Model file for the job. Use its own axes, mm. Face numbers are marked on the shaded views. A direction names the side the tool comes from. Round coordinates to 2 decimals unless told otherwise and drop trailing zeros. Loops run counter-clockwise (first coordinate to the right, second up) from the corner with the lowest first, then second, coordinate; pieces in that order, holes last. Notation, with made-up numbers: M -20.75,34.25 L 9.25,34.25 A24 ccw 9.25,62.25 Z; hole C -22,38 d9. An arc over 180 degrees is marked long. Use a Markdown table: item, result. Add a question column.
Item 1: Pin check, flat tips, straight feed: P1, Ø1, axis at x = 0.5, z = -1, coming from the +Y side; P2, Ø2, axis at y = 10, z = 0, coming from the +X side. Stop position of each tip, or through.
Item 2: Wall check: L1, parallel to Z at x = -0.55, y = 9.35; L2, parallel to Y at x = -0.8, z = 0.1; L3, parallel to X at y = 10.25, z = 0.4. Give the ranges that are in metal, low to high. Write a range as from..to.
Item 3: Saw through at D-D on x = -2.55. Write the cut outline in (y, z), then the cut area to 3 significant figures.
Item 4: Saw through at B-B on y = 8.65. Write the cut outline in (x, z), then the cut area to 3 significant figures.
Item 5: Saw through at C-C on z = 0.9. Write the cut outline in (x, y), then the cut area to 3 significant figures.
Item 6: Tool access for the marked faces 1 and 2: list every direction of +Z, -Z, +X, -X, +Y, -Y with a clear straight run to the whole face (end or side of a thin tool).
Item 7: Saw through at A-A on x = -0.8. Write the cut outline in (y, z), then the cut area to 3 significant figures.
```python
from build123d import *

# Parameters (mm, degrees)
SKETCH_1_W          = 30
SKETCH_1_H          = 20
EXTRUDE_1_DEPTH     = 20
CUT_EXTRUDE_3_REACH = 39.417
SKETCH_5_W          = 15
SKETCH_5_H          = 15
SCALE_1_SCALE       = 0.2


with BuildPart() as part:
    # 草圖1 → 填料-伸長1 (new body)
    with BuildSketch(Plane(origin=(0, 0, 0), x_dir=(1, 0, 0), z_dir=(0, 1, 0))):
        Rectangle(SKETCH_1_W, SKETCH_1_H)
    extrude(amount=EXTRUDE_1_DEPTH)

    # 除料-伸長3: up to this plane
    cut_extrude_3_end = Plane(origin=(7.5, 5, 2.5), z_dir=(-0.8017837257372732, -0.5345224838248487, -0.2672612419124243))
    # 草圖5 → 除料-伸長3 (cut, up to the surface)
    with BuildSketch(Plane(origin=(15, 0, 0), x_dir=(0, 0, -1), z_dir=(1, 0, 0)), mode=Mode.PRIVATE) as cut_extrude_3_sk1:
        with Locations((-2.5, 12.5)):
            Rectangle(SKETCH_5_W, SKETCH_5_H)
    cut_extrude_3_tool1 = split(extrude(cut_extrude_3_sk1.sketch, amount=-CUT_EXTRUDE_3_REACH, mode=Mode.PRIVATE), bisect_by=cut_extrude_3_end, keep=Keep.BOTH, mode=Mode.PRIVATE)
    add(cut_extrude_3_tool1.solids().sort_by_distance((15, 12.5, 2.5))[0], mode=Mode.SUBTRACT)


with BuildPart() as part_1:
    # 縮放比例1: scaled about (-2.551020408, 8.928571429, -0.918367347)
    add(part.part.scale(SCALE_1_SCALE).moved(Location((-2.040816326, 7.142857143, -0.734693878))))


solid = part_1.part
```
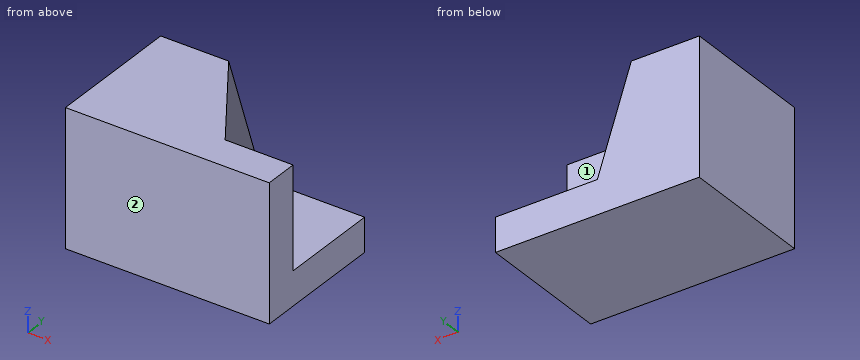
Entries:
| question | item | result |
|---|---|---|
| 1 | P1 | y = 8.14 |
| 1 | P2 | x = -1.11 |
| 2 | L1 | -2.73..-1.73 |
| 2 | L2 | 7.14..8.36 |
| 2 | L3 | -5.04..-2.16 |
| 3 | outline | M 7.14,-2.73 L 11.14,-2.73 L 11.14,-0.21 L 10.41,1.27 L 7.14,1.27 Z |
| 3 | area | 15.5 mm2 |
| 4 | outline | M -5.04,-2.73 L 0.96,-2.73 L 0.96,-1.73 L -0.38,-1.73 L -1.38,1.27 L -5.04,1.27 Z |
| 4 | area | 18.5 mm2 |
| 5 | outline | M -5.04,7.14 L 0.96,7.14 L 0.96,8.14 L -0.92,8.14 L -2.92,11.14 L -5.04,11.14 Z |
| 5 | area | 15.4 mm2 |
| 6 | face 1 | +Z, +X, +Y |
| 6 | face 2 | +Z, -Z, +X, -X, -Y |
| 7 | outline | M 7.14,-2.73 L 11.14,-2.73 L 11.14,-1.73 L 9.28,-1.73 L 8.14,0.54 L 8.14,1.27 L 7.14,1.27 Z |
| 7 | area | 8.30 mm2 |
